Autodesk Inventor part; units mm, degrees
ref_plane "YZ Plane" through (0, 0, 0) normal (1, 0, 0) x (0, 1, 0)
ref_plane "XZ Plane" through (0, 0, 0) normal (0, 1, 0) x (-1, 0, 0)
ref_plane "XY Plane" through (0, 0, 0) normal (0, 0, 1) x (1, 0, 0)
sketch "Sketch1" plane through (0, 0, 0) normal (0, 0, 1) x (1, 0, 0)
  line L0 (0, 12.6) -> (151.5, 12.6)
  arc A0 (151.5, -12.6) -> (151.5, 12.6) centre (151.5, 0) ccw
  line L1 (151.5, -12.6) -> (0, -12.6)
  arc A1 (0, 12.6) -> (0, -12.6) centre (0, 0) ccw
  circle A2 centre (0, 0) radius 7.5
  circle A3 centre (151.5, 0) radius 4.25
  dimension "d0" = 151.5
  dimension "d2" = 12.6
  dimension "d3" = 15
  dimension "d4" = 8.5
extrude "Extrusion1" add sketch "Sketch1" along normal blind 21.1
sketch "Sketch2" plane through (0, 0, 21.1) normal (0, 0, 1) x (1, 0, 0)
  circle A0 centre (0, 0) radius 7.5
  arc A1 (0, 12.6) -> (0, -12.6) centre (0, 0) ccw
  circle A2 centre (0, 0) radius 11
  dimension "d7" = 22
extrude "Extrusion2" cut sketch "Sketch2" against normal blind 7
sketch "Sketch6" plane through (0, 0, 21.1) normal (0, 0, 1) x (1, 0, 0)
  circle A0 centre (0, 0) radius 11
  arc A1 (0, 12.6) -> (0, -12.6) centre (0, 0) ccw
  circle A2 centre (0, 0) radius 17.5
  dimension "d25" = 35
extrude "Extrusion5" add sketch "Sketch6" against normal up to surface (21.1 mm away)
sketch "Sketch7" plane through (0, 0, 0) normal (0, 0, -1) x (-1, 0, 0)
  circle A0 centre (0, 0) radius 7.5
  circle A1 centre (0, 0) radius 11
extrude "Extrusion6" cut sketch "Sketch7" against normal blind 7
sketch "Sketch8" plane through (0, 0, 0) normal (0, 0, -1) x (-1, 0, 0)
  circle A0 centre (-151.5, 0) radius 4.25
  arc A1 (-151.5, 12.6) -> (-151.5, -12.6) centre (-151.5, 0) ccw
  line L0 (-143.9944, 0) -> (-147.7472, -6.5)
  line L1 (-147.7472, -6.5) -> (-155.2528, -6.5)
  line L2 (-155.2528, -6.5) -> (-159.0056, 0)
  line L3 (-159.0056, 0) -> (-155.2528, 6.5)
  line L4 (-155.2528, 6.5) -> (-147.7472, 6.5)
  line L5 (-147.7472, 6.5) -> (-143.9944, 0)
  dimension "d31" = 13
extrude "Extrusion7" cut sketch "Sketch8" against normal blind 8
fillet "Fillet1" radius 3.5 1 edges at (-7.5, 0, 14.1)
fillet "Fillet2" radius 3.5 1 edges at (-7.5, 0, 7)
properties part number "proximal thin arm"
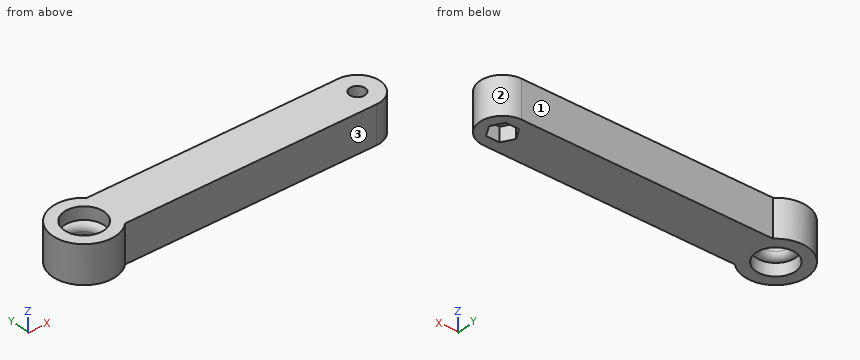
Geometry check sheet. Reference: the model listing, model coordinates, mm. Face numbers are marked on the shaded views. A direction names the side the tool comes from. Round coordinates to 2 decimals unless told otherwise and drop trailing zeros. Write each loop counter-clockwise with the first axis right and the second up, starting at its lowest first coordinate (ties: lowest second). Pieces come first, ordered by that corner, then holes. Notation, with made-up numbers: (-25, 77) -> (-12, 77) arc R21 cw to (-12, 86) -> close; hole circle Ø3 at (-29.5, -20.5). An arc over 180 degrees is marked (long way). Put each result on its own line as item: value.
1) Depth check by flat-ended pin: P1, Ø1, axis at x = 57.5, y = -8.5, coming from the -Z side; P2, Ø2, axis at y = 10.5, z = 4, coming from the -X side; P3, Ø17, axis at x = 0, y = 0, coming from the +Z side; P4, Ø4, axis at x = 150, z = 5, coming from the +Y side. Enter the tip coordinate at first touch or a pass-through.
Recorded:
P1: stops at z = 0
P2: stops at x = -14.7
P3: stops at z = 13.05
P4: stops at y = 12.6
2) Access from +Z, -Z, +X, -X, +Y, -Y to the whole of each face (thin tool, end or side, straight path). Record for the marked faces 1, 2 and 3.
Recorded:
face 1: +Z, -Z, +X, +Y
face 2: +Z, -Z, +X
face 3: +Z, -Z, +X, -Y
3) Thickness scan on probe 1 along Y at (x, z) = (0, 19.25); probe 2 along Y at (x, z) = (0, 10.65); probe 3 along X at (y, z) = (-2, 6). Record the ranges inside material, lowest first. Write a range as from..to.
Recorded:
probe 1: y = -17.5..-11, 11..17.5
probe 2: y = -17.5..-7.5, 7.5..17.5
probe 3: x = -17.39..-10.82, 10.82..145.15, 157.85..163.94
4) Cross-section at C-C, the plane y = -2. Give the number of separate pieces and of enclosed holes in the cut face, plus the area to 3 significant figures.
Recorded:
separate pieces: 3
enclosed holes: 0
area: 3,210 mm2
5) Cross-section at B-B, the plane x = 48. Enter the section's corners in (y, z), plus the area to 3 significant figures.
Recorded:
outline: (-12.6, 0) -> (12.6, 0) -> (12.6, 21.1) -> (-12.6, 21.1) -> close
area: 532 mm2
6) Cross-section at D-D, the plane y = -15. Enter the section's corners in (x, z).
Recorded:
outline: (-9.01, 0) -> (9.01, 0) -> (9.01, 21.1) -> (-9.01, 21.1) -> close
